Autodesk Fusion 360 part; units mm, degrees
sketch "Sketch1" plane through (0, 0, 0) normal (0, 0, 1) x (1, 0, 0)
  circle A0 centre (0, 0) radius 23
  dimension "d1" = 46
extrude "Extrude1" add sketch "Sketch1" along normal blind 10.2
sketch "Sketch2" plane through (0, 0, 0) normal (0, 0, 1) x (1, 0, 0)
  line L0 (-16.25, 4.6) -> (-14.6, 4.6)
  line L1 (-14.6, 4.6) -> (-17.9, 4.6)
  line L2 (-17.9, 4.6) -> (-17.9, -4.6)
  line L3 (-17.9, -4.6) -> (-14.6, -4.6)
  line L4 (-14.6, -4.6) -> (-14.6, 4.6)
  line L5 (14.6, 0) -> (14.6, 4.6)
  line L6 (14.6, 4.6) -> (17.9, 4.6)
  line L7 (17.9, 4.6) -> (14.6, 4.6)
  line L8 (14.6, 4.6) -> (14.6, -4.6)
  line L9 (14.6, -4.6) -> (17.9, -4.6)
  line L10 (17.9, -4.6) -> (17.9, 4.6)
  dimension "d6" = 1.65
  dimension "d7" = 3.3
  dimension "d8" = 9.2
  dimension "d10" = 14.6
  dimension "d11" = 3.3
  dimension "d12" = 3.3
  dimension "d13" = 9.2
extrude "Extrude2" add sketch "Sketch2" against normal blind 0.3
sketch "Sketch5" plane through (0, 0, 0) normal (0, 0, -1) x (1, 0, 0)
  line L0 (-14.6, -4.6) -> (-17.9, -4.6)
  line L1 (-17.9, -4.6) -> (-17.9, 4.6)
  line L2 (-17.9, 4.6) -> (-14.6, 4.6)
  line L3 (-14.6, 4.6) -> (-14.6, -4.6)
  line L4 (17.9, -4.6) -> (14.6, -4.6)
  line L5 (14.6, -4.6) -> (14.6, 4.6)
  line L6 (14.6, 4.6) -> (17.9, 4.6)
  line L7 (17.9, 4.6) -> (17.9, -4.6)
  circle A0 centre (0, 0) radius 23
  circle A1 centre (0, 0) radius 23
  line L8 (-17.9, 4.6) -> (-14.6, 4.6)
  line L9 (-14.6, 4.6) -> (-14.6, -4.6)
  line L10 (-14.6, -4.6) -> (-17.9, -4.6)
  line L11 (-17.9, -4.6) -> (-17.9, 4.6)
  line L12 (14.6, 4.6) -> (17.9, 4.6)
  line L13 (17.9, 4.6) -> (17.9, -4.6)
  line L14 (17.9, -4.6) -> (14.6, -4.6)
  line L15 (14.6, -4.6) -> (14.6, 4.6)
extrude "Extrude3" cut 1 faces at (-0.5729, -10.7119, 0) along direction (0, 0, 1) blind 4
sketch "Sketch6" plane through (0, 0, 4) normal (0, 0, -1) x (1, 0, 0)
  line L0 (-14.6, -4.6) -> (-17.9, -4.6)
  line L1 (-17.9, -4.6) -> (-17.9, 4.6)
  line L2 (-17.9, 4.6) -> (-14.6, 4.6)
  line L3 (-14.6, 4.6) -> (-14.6, -4.6)
  line L4 (17.9, -4.6) -> (14.6, -4.6)
  line L5 (14.6, -4.6) -> (14.6, 4.6)
  line L6 (14.6, 4.6) -> (17.9, 4.6)
  line L7 (17.9, 4.6) -> (17.9, -4.6)
  circle A0 centre (0, 0) radius 23
  line L8 (0, 0) -> (0, 11.6)
  line L9 (0, 0) -> (0, -11.5)
  line L10 (0, 11.6) -> (-15.75, 11.6)
  line L11 (0, 11.6) -> (15.75, 11.6)
  line L12 (0, -11.5) -> (15.75, -11.5)
  line L13 (0, -11.5) -> (-15.75, -11.5)
  circle A1 centre (-15.75, 11.6) radius 1.9
  circle A2 centre (15.4643, 11.6) radius 1.9
  circle A3 centre (-15.75, -11.5) radius 1.9
  circle A4 centre (15.75, -11.5) radius 1.9
  dimension "d18" = 11.6
  dimension "d19" = 11.5
  dimension "d20" = 15.75
  dimension "d21" = 15.75
  dimension "d22" = 15.75
  dimension "d23" = 15.75
  dimension "d24" = 3.8
  dimension "d25" = 3.8
  dimension "d26" = 3.8
  dimension "d27" = 3.8
extrude "Extrude4" add sketch "Sketch6" along normal blind 4 contours A1 | A2 | A4 | A3
extrude "Extrude5" add 2 faces at (-15.7, -1.5333, -0.3) (15.7, 1.5333, -0.3) along direction (0, 0, -1) blind 0.2
sketch "Sketch7" plane through (0, 0, 0) normal (0, 1, 0) x (1, 0, 0)
sketch "Sketch8" plane through (0, 0, 0) normal (0, 0, 1) x (1, 0, 0)
  line L0 (0, 0) -> (15, 0)
  line L1 (15, 0) -> (15, 15.5)
  line L2 (15, 15.5) -> (0, 15.5)
  line L3 (0, 15.5) -> (0, 0)
  dimension "d32" = 15
  dimension "d33" = 15.5
sketch "Sketch9" plane through (0, 0, -0.5) normal (0, 0, -1) x (1, 0, 0)
  line L0 (17.9, -4.6) -> (17.9, 4.6)
  line L1 (17.9, 4.6) -> (14.6, 4.6)
  line L2 (14.6, 4.6) -> (14.6, -4.6)
  line L3 (14.6, -4.6) -> (17.9, -4.6)
  line L4 (15, -15.5) -> (-15, -15.5)
  line L5 (-15, -15.5) -> (-15, 15.5)
  line L6 (-15, 15.5) -> (15, 15.5)
  line L7 (15, 15.5) -> (15, -15.5)
  line L8 (0, 0) -> (16, 0)
  dimension "d34" = 30
  dimension "d35" = 31
sketch "Sketch10" plane through (0, 0, 0) normal (0, 0, 1) x (1, 0, 0)
  line L0 (0, -23) -> (6, -23)
  line L1 (6, -23) -> (6, -14)
  line L2 (6, -14) -> (0, -14)
  line L3 (0, -14) -> (0, -23)
  line L4 (6, -14) -> (-6, -14)
  line L5 (-6, -14) -> (-6, -23)
  line L6 (-6, -23) -> (6, -23)
  line L7 (6, -23) -> (6, -14)
  circle A0 centre (0, 0) radius 23
  dimension "d36" = 6
  dimension "d37" = 12
extrude "Extrude6" add sketch "Sketch10" along normal blind 4 contours L3 L4 L5 A0 | L1 L2 L3 L4 L7 A0
sketch "Sketch11" plane through (0, 0, -0.5) normal (0, 0, -1) x (1, 0, 0)
  line L0 (0, 23) -> (0, 15.5)
sketch "Sketch12" plane through (0, 0, 0) normal (1, 0, 0) x (0, 1, 0)
sketch "Sketch13" plane through (0, 0, -0.5) normal (0, 0, -1) x (1, 0, 0)
  line L0 (0, 0) -> (-14.6, 0)
  line L1 (-14.6, 0) -> (-17.9, 0)
  line L2 (-14.6, 4.6) -> (-17.9, 4.6)
  line L3 (-17.9, 4.6) -> (-17.9, -4.6)
  line L4 (-17.9, -4.6) -> (-14.6, -4.6)
  line L5 (-14.6, -4.6) -> (-14.6, 4.6)
sketch "Sketch14" plane through (17.9, 0, 0) normal (1, 0, 0) x (0, 1, 0)
  line L0 (-4.6, 4) -> (-4.6, -0.5)
  line L1 (-4.6, -0.5) -> (4.6, -0.5)
  line L2 (4.6, -0.5) -> (4.6, 4)
  line L3 (4.6, 4) -> (-4.6, 4)
ref_plane "WorkPlane1" through (0, 0, 0) normal (1, 0, 0) x (0, 1, 0)
ref_plane "WorkPlane2" through (0, 0, 0) normal (0, 1, 0) x (0, 0, 1)
sketch "Sketch15" plane through (0, 0, 10.2) normal (0, 0, 1) x (-1, 0, 0)
  circle A0 centre (0, 0) radius 23
  circle A1 centre (0, 0) radius 18.375
  dimension "d42" = 36.75
extrude "Extrude7" cut sketch "Sketch15" against normal blind 0.1 contours A1
equation "d6 = ( 3.3 / 2 ) * 1 mm"
equation "d20 = ( 31.5 / 2 ) * 1 mm"
equation "d21 = ( 31.5 / 2 ) * 1 mm"
equation "d22 = ( 31.5 / 2 ) * 1 mm"
equation "d23 = ( 31.5 / 2 ) * 1 mm"
Input: part model. Units: mm. Frame: model coordinates. A direction names the side the tool comes from. Coordinates: 2 decimals unless noted, no trailing zeros. Loops run counter-clockwise (first coordinate to the right, second up) from the corner with the lowest first, then second, coordinate; pieces in that order, holes last. Notation, with made-up numbers: (-2, 50) -> (27, 50) arc R9 cw to (27, 57) -> close; hole circle Ø6 at (-39, -18). An arc over 180 degrees is marked (long way). Write item = value, one per line. Start each with the question number.
Item 1: Mould query, pull axis Y, two halves, no side actions, for faces 1 (the face through (-17.9, 0, 2)), 2 (the face through (-2.994, -22.804, 7.295)), 3 (the face through (-16, 4.6, 2)). Classes: pulls with the +Y half, pulls with the -Y half, needs draft (parallel to the pull), parting line crosses it, or undercut.
Item 2: Cut plane A-A, the plane x = 0. Return loops of the section in (y, z) (3 decimals).
Item 3: Material intervals for line 1 (X direction, y = 0, z = 10.15) (3 decimals); line 2 (Z direction, x = -9.5, y = 19.5); line 3 (Z direction, x = 4, y = -5), sorted ascending.
Item 4: Reachability of faces 4 (the face through (16, 11, 0)), 5 (the face through (14.6, 0, 2)), 6 (the face through (17.9, 0, 2)), 7 (the face through (-16, -4.6, 2)), 8 (the face through (-6, -18, 2)) from +Z, -Z, +X, -X, +Y, -Y: full face, straight path, thin tool, end or side. Return the list, or none.
Item 5: Cut plane D-D, the plane x = 15.75. Return loops of the section in (y, z), plus the area to 3 significant figures.
Item 6: First-contact query: P1, Ø4, axis at x = -15.5, y = -12.5, coming from the -Z side; P2, Ø1.3, axis at y = 2, z = 2, coming from the -X side; P3, Ø18.5, axis at x = 3.5, y = -5, coming from the +Z side. Flat tips, straight axial feed; report the tip coordinate or a pass-through.
Item 7: Cut plane C-C, the plane z = 8. Return loops of the section in (x, y), plus the area to 3 significant figures.
Item 8: Cut plane B-B, the plane y = 0. Return loops of the section in (x, z) (3 decimals).
Ans:
q1.face_1 = needs draft
q1.face_2 = parting line crosses it
q1.face_3 = undercut
q2.outline = (-23, 0) -> (-14, 0) -> (-14, 4) -> (23, 4) -> (23, 10.2) -> (18.375, 10.2) -> (18.375, 10.1) -> (-18.375, 10.1) -> (-18.375, 10.2) -> (-23, 10.2) -> close
q3.line_1 = -23 to -18.375, 18.375 to 23
q3.line_2 = 4 to 10.2
q3.line_3 = 4 to 10.1
q4.face_4 = -Z, +X, -X, +Y
q4.face_5 = -Z
q4.face_6 = -Z, +X, +Y, -Y
q4.face_7 = -Z, +X, -X
q4.face_8 = -Z, -X, +Y, -Y
q5.outline = (-16.76, 4) -> (-13.48, 4) -> (-13.48, 0) -> (-9.72, 0) -> (-9.72, 4) -> (-4.6, 4) -> (-4.6, -0.5) -> (4.6, -0.5) -> (4.6, 4) -> (9.6, 4) -> (9.6, 0) -> (13.4, 0) -> (13.4, 4) -> (16.76, 4) -> (16.76, 10.2) -> (9.46, 10.2) -> (9.46, 10.1) -> (-9.46, 10.1) -> (-9.46, 10.2) -> (-16.76, 10.2) -> close
q5.area = 278 mm²
q6.P1 = 0
q6.P2 = -17.9
q6.P3 = 10.1
q7.outline = circle Ø46 at (0, 0)
q7.area = 1,660 mm²
q8.outline = (-23, 4) -> (-17.9, 4) -> (-17.9, -0.5) -> (-14.6, -0.5) -> (-14.6, 4) -> (14.6, 4) -> (14.6, -0.5) -> (17.9, -0.5) -> (17.9, 4) -> (23, 4) -> (23, 10.2) -> (18.375, 10.2) -> (18.375, 10.1) -> (-18.375, 10.1) -> (-18.375, 10.2) -> (-23, 10.2) -> close
